Build history of the part. All positions in model axes, mm. A direction names the side the tool comes from. Give positions to 0.01 mm unless a question says otherwise; leave off trailing zeros. Write each loop counter-clockwise with the first axis right and the second up, starting at its lowest first coordinate (ties: lowest second). Pieces come first, ordered by that corner, then holes. Notation, with made-up numbers: (48.25, -35) -> (55.25, -35) arc R24 cw to (55.25, -11) -> close; hole circle Ø1 at (29.25, -4). An arc over 180 degrees is marked (long way). Write item = value, one per line. Start each with the question number.
Q1. Saw through at D-D, the plane x = -6.5. List the corners of the cut face in (y, z).
Q2. Wall check: line 1 (Y direction, x = 21.7, z = 0.6); line 2 (Y direction, x = -23, z = 0.5). Give the ranges that are in metal, low to high.
Q3. Saw through at B-B, the plane z = 1.6. Give the number of separate pieces and of enclosed holes in the cut face, then the cut area to 3 significant figures.
Q4. Mould opens along X. For faces 3 (the face through (-20.73, -22.97, 1.29)), 4 (the face through (0, 29, 1)), 5 (the face through (26, -27, 1)) say: pulls with the +X half, pulls with the -X half, needs draft (parallel to the pull), parting line crosses it, or undercut.
Q5. Drop flat-ended pins along their axis: P1, Ø3, axis at x = -21.7, y = -21.7, coming from the +Z side; P2, Ø0.8, axis at x = 1.5, z = 1, coming from the -Y side. Give the stop position or say it passes through.
Q6. Tool access for faces 1 (the face through (16, -25.5, 1.3)), 2 (the face through (22, -29, 1)): list every direction of +Z, -Z, +X, -X, +Y, -Y with a clear straight run to the whole face (end or side of a thin tool).
Q7. Saw through at A-A, the plane y = 21.7. List the corners of the cut face in (x, z), then the cut area to 3 significant figures.
Autodesk Inventor part; units mm, degrees
ref_plane "YZ Plane" through (0, 0, 0) normal (1, 0, 0) x (0, 1, 0)
ref_plane "XZ Plane" through (0, 0, 0) normal (0, 1, 0) x (-1, 0, 0)
ref_plane "XY Plane" through (0, 0, 0) normal (0, 0, 1) x (1, 0, 0)
sketch "Sketch1" plane through (0, 0, 0) normal (0, 0, 1) x (1, 0, 0)
  line L0 (29, 29) -> (-29, 29)
  line L1 (-29, 29) -> (-29, -29)
  line L2 (-29, -29) -> (29, -29)
  line L3 (29, -29) -> (29, 29)
  line L4 (29, 29) -> (-29, -29) construction
  line L5 (-29, 29) -> (29, -29) construction
  line L6 (21.7, -21.7) -> (-21.7, -21.7) construction
  line L7 (-21.7, -21.7) -> (-21.7, 21.7) construction
  line L8 (-21.7, 21.7) -> (21.7, 21.7) construction
  line L9 (21.7, 21.7) -> (21.7, -21.7) construction
  line L10 (21.7, -21.7) -> (-21.7, 21.7) construction
  line L11 (-21.7, -21.7) -> (21.7, 21.7) construction
  line L12 (-12.5, -36) -> (12.5, -36)
  line L13 (12.5, -36) -> (12.5, -22)
  line L14 (12.5, -22) -> (-12.5, -22)
  line L15 (-12.5, -22) -> (-12.5, -36)
  line L16 (-12.5, -36) -> (12.5, -22) construction
  line L17 (12.5, -36) -> (-12.5, -22) construction
  point P0 (0, 0)
  point P1 (0, -29)
  dimension "d0" = 58
  dimension "d1" = 58
  dimension "d7" = 43.4
  dimension "d15" = 25
  dimension "d16" = 14
extrude "Extrusion1" add sketch "Sketch1" along normal blind 2.55 contours L3 L2 L13 L14 L15 L1 L0 | L2 L15 L14 L13
chamfer "Chamfer1" distance 5 angle 45 4 edges at (29, 29, 1.275) (-29, 29, 1.275) (-29, -29, 1.275) (29, -29, 1.275)
hole "Hole1" at (-21.7, 21.7, 0) at (-21.7, -21.7, 0) at (21.7, -21.7, 0) at (21.7, 21.7, 0) direction (0, 0, 1) diameter 3.2 end through all
extrude "Extrusion2" cut sketch "Sketch1" along normal up to next contours L13 L12 L15 L2 | L2 L15 L14 L13
chamfer "Chamfer2" distance 7 angle 45 2 edges at (-12.5, -29, 1.275) (12.5, -29, 1.275)
sketch "Sketch2" plane through (0, 0, 2.55) normal (0, 0, 1) x (1, 0, 0)
  line L0 (19.5, -29) -> (12.5, -22)
  line L1 (19.5, -29) -> (24, -29)
  line L2 (29, -24) -> (24, -29)
  line L3 (29, -24) -> (29, 24)
  line L4 (24, 29) -> (29, 24)
  line L5 (24, 29) -> (-24, 29)
  line L6 (-29, 24) -> (-24, 29)
  line L7 (-29, 24) -> (-29, -24)
  line L8 (-24, -29) -> (-29, -24)
  line L9 (-24, -29) -> (-19.5, -29)
  line L10 (-12.5, -22) -> (-19.5, -29)
  line L11 (-12.5, -22) -> (12.5, -22)
  circle A0 centre (21.7, 21.7) radius 1.6
  circle A1 centre (-21.7, -21.7) radius 1.6
  circle A2 centre (-21.7, 21.7) radius 1.6
  circle A3 centre (21.7, -21.7) radius 1.6
  point P0 (0, 0)
properties part number "compactActiveLoad_BottomCover"
Report:
q1.outline = (-22, 0) -> (29, 0) -> (29, 2.55) -> (-22, 2.55) -> close
q2.line_1 = -29 to -23.3, -20.1 to 20.1, 23.3 to 29
q2.line_2 = -29 to -22.63, -20.77 to 20.77, 22.63 to 29
q3.separate_pieces = 1
q3.enclosed_holes = 4
q3.area = 3,060 mm2
q4.face_3 = undercut
q4.face_4 = needs draft
q4.face_5 = pulls with the +X half
q5.P1 = through
q5.P2 = -22
q6.face_1 = +Z, -Z, -Y
q6.face_2 = +Z, -Z, +X, -X, -Y
q7.outline = (-29, 0) -> (-23.3, 0) -> (-23.3, 2.55) -> (-29, 2.55) -> close; (-20.1, 0) -> (20.1, 0) -> (20.1, 2.55) -> (-20.1, 2.55) -> close; (23.3, 0) -> (29, 0) -> (29, 2.55) -> (23.3, 2.55) -> close
q7.area = 132 mm2
